Here's how the part is built. I have some questions about the finished solid (model axes, mm). A direction names the side the tool comes from. Round coordinates to 2 decimals unless told otherwise and drop trailing zeros. Loops run counter-clockwise (first coordinate to the right, second up) from the corner with the lowest first, then second, coordinate; pieces in that order, holes last. Notation, with made-up numbers: M 42,-40 L 64,-40 A21 cw 64,-20 Z; hole C 41,19.5 d1. An arc over 180 degrees is marked long. Answer as a JSON object with one key per item and string values.
from build123d import *

# Parameters (mm, degrees)
SKETCH_4_R          = 26
SKETCH_4_R_2        = 7.5
SKETCH_4_R_3        = 5
EXTRUDE_2_DEPTH     = 10
SKETCH_4_4_R        = 5
SKETCH_4_4_R_2      = 2
EXTRUDE_3_DEPTH     = 5
SKETCH_5_R          = 12.5
CUT_EXTRUDE_3_DEPTH = 5


with BuildPart() as part:
    # Sketch 4 → Extrude 2 (new body)
    with BuildSketch(Plane.XY):
        Circle(SKETCH_4_R)
        Circle(SKETCH_4_R_2, mode=Mode.SUBTRACT)
        with Locations((-18, 0)):
            Circle(SKETCH_4_R_3, mode=Mode.SUBTRACT)
        with Locations((18, 0)):
            Circle(SKETCH_4_R_3, mode=Mode.SUBTRACT)
    extrude(amount=EXTRUDE_2_DEPTH)

    # Sketch 4_4 → Extrude 3 (add)
    # profile 1 of 2: a face of its own
    with BuildSketch(Plane.XY):
        with Locations((-18, 0)):
            Circle(SKETCH_4_4_R)
        with Locations((-18, 0)):
            Circle(SKETCH_4_4_R_2, mode=Mode.SUBTRACT)
    # profile 2 of 2: a face of its own
    with BuildSketch(Plane.XY):
        with Locations((18, 0)):
            Circle(SKETCH_4_4_R)
        with Locations((18, 0)):
            Circle(SKETCH_4_4_R_2, mode=Mode.SUBTRACT)
    extrude(amount=EXTRUDE_3_DEPTH)

    # Sketch 5 → Cut-Extrude 3 (cut)
    with BuildSketch(Plane.XY.offset(10)):
        Circle(SKETCH_5_R)
    extrude(amount=-CUT_EXTRUDE_3_DEPTH, mode=Mode.SUBTRACT)


solid = part.part
Item 1: I want a section at A-A on x = 0. List the corners of the cut face in (y, z) for me, plus the area to 3 significant figures.
Solution:
{"outline": "M -26,0 L -7.5,0 L -7.5,5 L -12.5,5 L -12.5,10 L -26,10 Z; M 7.5,0 L 26,0 L 26,10 L 12.5,10 L 12.5,5 L 7.5,5 Z", "area": "320 mm2"}
Item 2: For P1, Ø4.5, axis at x = -18, y = 0, coming from the +Z side; P2, Ø4, axis at y = 10.5, z = 4, coming from the -X side; P3, Ø3, axis at y = 11, z = 4.5, coming from the -X side, each with a flat end and sliding along its axis, tell me the tip position at first contact or that it passes through.
Solution:
{"P1": "stops at z = 5", "P2": "stops at x = -24.57", "P3": "stops at x = -24.2"}
Item 3: I want a section at D-D on x = -18. List the corners of the cut face in (y, z) for me.
Solution:
{"outline": "M -18.76,0 L -2,0 L -2,5 L -5,5 L -5,10 L -18.76,10 Z; M 2,0 L 18.76,0 L 18.76,10 L 5,10 L 5,5 L 2,5 Z"}
Item 4: I want a section at C-C on z = 1.75. List the corners of the cut face in (x, y) for me, plus the area to 3 significant figures.
Solution:
{"outline": "C 0,0 d52; hole C -18,0 d4; hole C 0,0 d15; hole C 18,0 d4", "area": "1,920 mm2"}
Item 5: I want a section at B-B on y = 0. List the corners of the cut face in (x, z) for me.
Solution:
{"outline": "M -26,0 L -20,0 L -20,5 L -23,5 L -23,10 L -26,10 Z; M -16,0 L -7.5,0 L -7.5,5 L -12.5,5 L -12.5,10 L -13,10 L -13,5 L -16,5 Z; M 7.5,0 L 16,0 L 16,5 L 13,5 L 13,10 L 12.5,10 L 12.5,5 L 7.5,5 Z; M 20,0 L 26,0 L 26,10 L 23,10 L 23,5 L 20,5 Z"}
Item 6: For faces 1 (the face through (-18.1, -2.2, 5)), 2 (the face through (-19.6, -1.2, 2.5)), which set-ups out of +Z, -Z, +X, -X, +Y, -Y let a thin tool reach every point of the face, with its end or its side?
Solution:
{"face 1": "+Z", "face 2": "+Z, -Z"}
Item 7: If I drill on L1, parallel to Y at x = 0, z = 8.55; L2, parallel to Y at x = 10, z = 8; L3, parallel to Z at x = 8.5, y = 4, over which ranges is the centre line in solid material (lowest first)? Write a range as from..to.
Solution:
{"L1": "y = -26..-12.5, 12.5..26", "L2": "y = -24..-7.5, 7.5..24", "L3": "z = 0..5"}
Item 8: We'd pull the mould along X, two halves only. Please class faces 3 (the face through (-20.633, -15.821, 4.93)), 4 (the face through (16.4, -1.2, 2.5)), 5 (the face through (-7.493, 0.33, 2.465)), 6 (the face through (-6.1, -11.2, 10)): +X half, -X half, draft (parallel to the pull), parting line (faces both ways), or undercut.
Solution:
{"face 3": "parting line", "face 4": "undercut", "face 5": "undercut", "face 6": "draft"}
